```python
from build123d import *

# Parameters (mm, degrees)
EXTRUDE_1_DEPTH = 3
SKETCH_1_4_R    = 2.5
EXTRUDE_3_DEPTH = 15


with BuildPart() as part:
    # Sketch 1 → Extrude 1 (new body)
    with BuildSketch(Plane.XY):
        with BuildLine():
            Line((0, 5), (25, 5))
            ThreePointArc((25, 5), (30, 0), (25, -5))
            Line((25, -5), (0, -5))
            ThreePointArc((0, -5), (-5, 0), (0, 5))
        make_face()
    extrude(amount=EXTRUDE_1_DEPTH)

    # Sketch 1_4 → Extrude 3 (add)
    with BuildSketch(Plane.XY):
        with Locations((25, 0)):
            Circle(SKETCH_1_4_R)
    extrude(amount=EXTRUDE_3_DEPTH)


solid = part.part
```
Input: part model. Units: mm. Frame: model coordinates. A direction names the side the tool comes from. Round coordinates to 2 decimals unless told otherwise and drop trailing zeros. Loops run counter-clockwise (first coordinate to the right, second up) from the corner with the lowest first, then second, coordinate; pieces in that order, holes last.
1) Section query C-C on z = 10.25. Return the cut outline in (x, y), plus the area to 3 significant figures.
Ans:
outline: circle Ø5 at (25, 0)
area: 19.6 mm2
2) Section query B-B on x = 27. Return the cut outline in (y, z).
Ans:
outline: (-4.58, 0) - (4.58, 0) - (4.58, 3) - (1.5, 3) - (1.5, 15) - (-1.5, 15) - (-1.5, 3) - (-4.58, 3) - close
3) Section query A-A on y = 0. Return the cut outline in (x, z), plus the area to 3 significant figures.
Ans:
outline: (-5, 0) - (30, 0) - (30, 3) - (27.5, 3) - (27.5, 15) - (22.5, 15) - (22.5, 3) - (-5, 3) - close
area: 165 mm2
4) Set-up query: faces 1 (the flat face through (13, -5, 1)), 2 (the cylindrical face through (22.5, 0.1, 8.9)). Return all of +Z, -Z, +X, -X, +Y, -Y with unobstructed straight access to the full face (end or side cutting, diameter ignored); none if empty.
Ans:
face 1: +Z, -Z, +X, -X, -Y
face 2: +Z
5) Pin query (flat end, axial travel): pin 1 (4 mm diameter, centred on y = 2.5, z = 3, fed in from +X); pin 2 (5 mm diameter, centred on x = 17, y = 1.5, fed in from +Z); pin 3 (5 mm diameter, centred on y = -0.5, z = 7, fed in from +X). Return the tip coordinate at first contact, or that it passes through.
Ans:
pin 1: stops at x = 29.97
pin 2: stops at z = 3
pin 3: stops at x = 27.5
6) Section query D-D on y = 4. Return the cut outline in (x, z), plus the area to 3 significant figures.
Ans:
outline: (-3, 0) - (28, 0) - (28, 3) - (-3, 3) - close
area: 93.0 mm2
7) Material intervals for line 1 (Z direction, x = 19.5, y = -0.5); line 2 (X direction, y = -0.25, z = 0.75); line 3 (X direction, y = 0, z = 6.5), sorted ascending.
Ans:
line 1: z = 0 to 3
line 2: x = -4.99 to 29.99
line 3: x = 22.5 to 27.5
